The drawing under review shows one solid part. Ordinate dimensions are in mm from its lowest x, y, z. Coordinates: 2 decimals unless noted, no trailing zeros. Write each loop counter-clockwise with the first axis right and the second up, starting at its lowest first coordinate (ties: lowest second). Pieces come first, ordered by that corner, then holes.
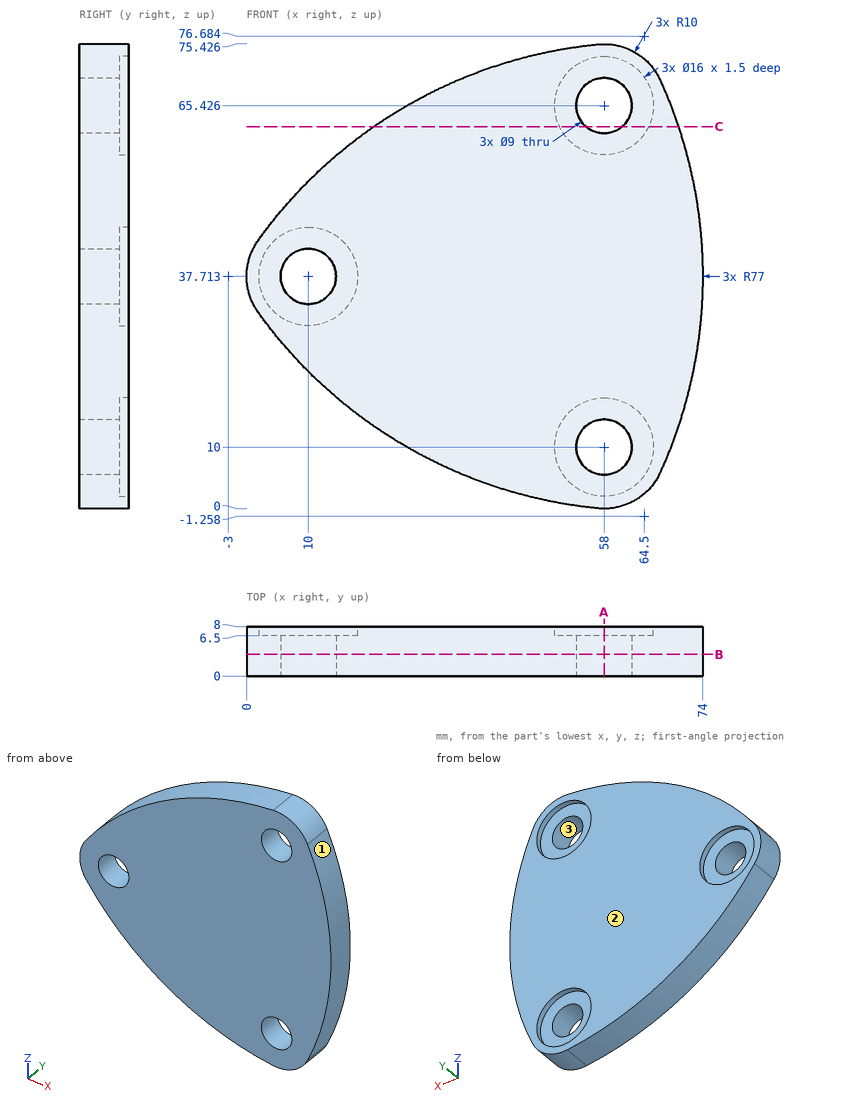
Q1. Add section C-C (z = 62). State the section outline as (x, y) points.
Ans:
outline: (20.6, 0) - (55.08, 0) - (55.08, 6.5) - (50.77, 6.5) - (50.77, 8) - (20.6, 8) - close; (60.92, 0) - (70.07, 0) - (70.07, 8) - (65.23, 8) - (65.23, 6.5) - (60.92, 6.5) - close
Q2. Add section A-A (x = 58). State the section outline as (y, z) points (1 decimal).
Ans:
outline: (0, 0) - (8, 0) - (8, 2) - (6.5, 2) - (6.5, 5.5) - (0, 5.5) - close; (0, 14.5) - (6.5, 14.5) - (6.5, 18) - (8, 18) - (8, 57.4) - (6.5, 57.4) - (6.5, 60.9) - (0, 60.9) - close; (0, 69.9) - (6.5, 69.9) - (6.5, 73.4) - (8, 73.4) - (8, 75.4) - (0, 75.4) - close
Q3. For probe 1 along X at (y, z) = (3.5, 37.5) (1 decimal); probe 2 along Z at (x, y) = (58, 5) (1 decimal); probe 3 along Y at (x, z) = (57, 4), list the stretches that pass through material, from the lowest coordinate up.
Ans:
probe 1: x = 0 to 5.5, 14.5 to 74
probe 2: z = 0 to 5.5, 14.5 to 60.9, 69.9 to 75.4
probe 3: y = 0 to 6.5
Q4. Draft analysis for pull direction Z (two halves, no side actions). For the marked faces 1, 2 and 3, state which applies: +Z half, -Z half, draft (parallel to the pull), parting line (faces both ways), or undercut.
Ans:
face 1: parting line
face 2: draft
face 3: undercut
Q5. Clearance check with flat-ended pins moving along their axes: pin 1 Ø13 at (x, z) = (11, 41.5) entering from +Y; pin 2 Ø2 at (x, y) = (31, 5) entering from -Z; pin 3 Ø3 at (y, z) = (7, 19) entering from +X; pin 4 Ø7 at (x, z) = (58, 10) entering from +Y. State where each tip first meets the part, or that it passes through.
Ans:
pin 1: stops at y = 8
pin 2: stops at z = 6.88
pin 3: stops at x = 72.05
pin 4: passes through
Q6. Add section B-B (y = 3.5). State the section outline as (x, z) points (1 decimal), then the cut area to 3 significant figures.
Ans:
outline: (1.9, 31.9) arc R77 ccw to (57, 0) arc R10 ccw to (67.1, 5.9) arc R77 ccw to (67.1, 69.6) arc R10 ccw to (57, 75.4) arc R77 ccw to (1.9, 43.5) arc R10 ccw to start; hole circle Ø9 at (10, 37.7); hole circle Ø9 at (58, 10); hole circle Ø9 at (58, 65.4)
area: 3,840 mm2
